from build123d import *

# Parameters (mm, degrees)
F0_R     = 2.413
F1_DEPTH = 7.62
F2_R     = 7.62
F2_R_2   = 1.27
F3_DEPTH = 2.794


with BuildPart() as f1:
    # F0 (on Top) → F1 (new body)
    with BuildSketch(Plane.XY):
        Circle(F0_R)
    extrude(amount=F1_DEPTH)

    # F2 (on face) → F3 (join)
    with BuildSketch(Plane.XY.offset(7.62)):
        Circle(F2_R)
        with Locations((-4.341766, -2.50672)):
            Circle(F2_R_2, mode=Mode.SUBTRACT)
        with Locations((0, -5.013439)):
            Circle(F2_R_2, mode=Mode.SUBTRACT)
        with Locations((4.341766, -2.50672)):
            Circle(F2_R_2, mode=Mode.SUBTRACT)
        with Locations((-4.341766, 2.50672)):
            Circle(F2_R_2, mode=Mode.SUBTRACT)
        with Locations((4.341766, 2.50672)):
            Circle(F2_R_2, mode=Mode.SUBTRACT)
        with Locations((0, 5.013439)):
            Circle(F2_R_2, mode=Mode.SUBTRACT)
    extrude(amount=F3_DEPTH)


solid = f1.part
Geometry: final body of the model. Coordinates: model frame, mm. A direction names the side the tool comes from. Round coordinates to 2 decimals unless told otherwise and drop trailing zeros. Loops run counter-clockwise (first coordinate to the right, second up) from the corner with the lowest first, then second, coordinate; pieces in that order, holes last.
Q1. Pull-direction query (X, two-part tool) for faces 1 (the cylindrical face through (-5.35, -3.28, 9)), 2 (the flat face through (0, 0, 10.414)), 3 (the cylindrical face through (-1.65, -7.44, 9)); classes: released by +X, released by -X, zero draft, split by the parting line, or undercut.
Q2. Material intervals for L1, parallel to Y at x = 5.5, z = 9.75; L2, parallel to Y at x = 0, z = 8.3; L3, parallel to Z at x = 1.5, y = 4.75, sorted ascending.
Q3. Section C-C on z = 8.25. Return loops of the section in (x, y).
Q4. Section A-A on x = 0. Return loops of the section in (y, z), plus the area to 3 significant figures.
Q5. Section B-B on y = 0. Return loops of the section in (x, z), plus the area to 3 significant figures.
Q6. Section D-D on y = -2. Return loops of the section in (x, z), plus the area to 3 significant figures.
Q7. Pin query (flat end, axial travel): P1, Ø4, axis at x = -4.34, y = -2.51, coming from the -Z side; P2, Ø2, axis at x = 2.5, z = 8, coming from the +Y side. Return the tip coordinate at first contact, or that it passes through.
Q8. Access query for faces 4 (the cylindrical face through (-5.278, 3.365, 8.997)), 5 (the cylindrical face through (-1.915, -1.468, 3.757)). Directions: +Z, -Z, +X, -X, +Y, -Y. A direction counts if a zero-diameter tool reaches every point of the face in a straight line with its end or side. Return the directions, or none.
Evaluation:
1. face 1: undercut
1. face 2: zero draft
1. face 3: split by the parting line
2. L1: y = -5.27 to -3.03, -1.99 to 1.99, 3.03 to 5.27
2. L2: y = -7.62 to -6.28, -3.74 to 3.74, 6.28 to 7.62
2. L3: z = 7.62 to 10.41
3. outline: circle Ø15.24 at (0, 0); hole circle Ø2.54 at (-4.34, -2.51); hole circle Ø2.54 at (-4.34, 2.51); hole circle Ø2.54 at (0, -5.01); hole circle Ø2.54 at (0, 5.01); hole circle Ø2.54 at (4.34, -2.51); hole circle Ø2.54 at (4.34, 2.51)
4. outline: (-7.62, 7.62) - (-6.28, 7.62) - (-6.28, 10.41) - (-7.62, 10.41) - close; (-3.74, 7.62) - (-2.41, 7.62) - (-2.41, 0) - (2.41, 0) - (2.41, 7.62) - (3.74, 7.62) - (3.74, 10.41) - (-3.74, 10.41) - close; (6.28, 7.62) - (7.62, 7.62) - (7.62, 10.41) - (6.28, 10.41) - close
4. area: 65.2 mm2
5. outline: (-7.62, 7.62) - (-2.41, 7.62) - (-2.41, 0) - (2.41, 0) - (2.41, 7.62) - (7.62, 7.62) - (7.62, 10.41) - (-7.62, 10.41) - close
5. area: 79.4 mm2
6. outline: (-7.35, 7.62) - (-5.51, 7.62) - (-5.51, 10.41) - (-7.35, 10.41) - close; (-3.18, 7.62) - (-1.35, 7.62) - (-1.35, 0) - (1.35, 0) - (1.35, 7.62) - (3.18, 7.62) - (3.18, 10.41) - (-3.18, 10.41) - close; (5.51, 7.62) - (7.35, 7.62) - (7.35, 10.41) - (5.51, 10.41) - close
6. area: 48.6 mm2
7. P1: stops at z = 7.62
7. P2: stops at y = 7.47
8. face 4: +Z, -Z
8. face 5: -Z
